Model file for the job. Use its own axes, mm. A direction names the side the tool comes from. Give positions to 0.01 mm unless a question says otherwise; leave off trailing zeros. Loops run counter-clockwise (first coordinate to the right, second up) from the corner with the lowest first, then second, coordinate; pieces in that order, holes last. Notation, with made-up numbers: (88.5, 11.5) - (112.5, 11.5) arc R31 cw to (112.5, 39.5) - close; hole circle Ø8 at (-14.5, 21.25). An arc over 180 degrees is marked (long way). Use a Markdown table: item, result.
Autodesk Inventor part; units mm, degrees
ref_plane "YZ Plane" through (0, 0, 0) normal (1, 0, 0) x (0, 1, 0)
ref_plane "XZ Plane" through (0, 0, 0) normal (0, 1, 0) x (-1, 0, 0)
ref_plane "XY Plane" through (0, 0, 0) normal (0, 0, 1) x (1, 0, 0)
sketch "Sketch1" plane through (0, 0, 0) normal (1, 0, 0) x (0, 1, 0)
  line L0 (0, 0) -> (-78.6, 0)
  line L1 (-78.6, 0) -> (-78.6, -45)
  line L2 (-78.6, -45) -> (0, -45)
  line L3 (0, -45) -> (0, 0)
  dimension "d0" = 78.6
  dimension "d1" = 45
extrude "Extrusion1" add sketch "Sketch1" along normal blind 20
sketch "Sketch2" plane through (20, 0, 0) normal (1, 0, 0) x (0, 0, -1)
  circle A0 centre (22.5, -27.8) radius 17.5
  line L0 (45, -78.6) -> (45, 0)
  line L1 (0, -78.6) -> (45, -78.6)
  point P0 (0, 0)
  dimension "d4" = 35
  dimension "d5" = 22.5
  dimension "d6" = 50.8
extrude "Extrusion2" add sketch "Sketch2" along normal blind 10
sketch "Sketch3" plane through (30, -27.8, -22.5) normal (1, 0, 0) x (0, 0, -1)
  circle A0 centre (0, 0) radius 3
  point P0 (-22.5, 27.8)
  dimension "d9" = 6
extrude "Extrusion3" add sketch "Sketch3" along normal blind 44
fillet "Fillet1" radius 5 2 edges at (10, 0, 0) (10, 0, -45)
sketch "Sketch4" plane through (0, 0, -5) normal (0, 1, 0) x (1, 0, 0)
  line L0 (6.488, 30) -> (2.488, 30)
  line L1 (2.488, 30) -> (2.488, 26)
  line L2 (2.488, 26) -> (6.488, 26)
  line L3 (6.488, 26) -> (6.488, 30)
  line L4 (6.488, 9) -> (2.488, 9)
  line L5 (2.488, 9) -> (2.488, 5)
  line L6 (2.488, 5) -> (6.488, 5)
  line L7 (6.488, 5) -> (6.488, 9)
  line L8 (0, 35) -> (20, 35)
  line L9 (20, 0) -> (0, 0)
  point P0 (0, -5)
  dimension "d13" = 4
  dimension "d14" = 4
  dimension "d15" = 4
  dimension "d16" = 4
  dimension "d17" = 5
  dimension "d18" = 9
extrude "Extrusion4" add sketch "Sketch4" along normal blind 5
chamfer "Chamfer1" distance 2 angle 45 1 edges at (30, -27.8, -5)
fillet "Fillet2" radius 5 5 edges at (20, -1.4645, -1.4645) (20, -41.8, 0) (20, -1.4645, -43.5355) (20, -41.8, -45) (20, 0, -22.5)
fillet "Fillet3" radius 2 1 edges at (74, -27.8, -19.5)
sketch "Sketch5" plane through (30, -27.8, -22.5) normal (1, 0, 0) x (0, 0, -1)
  point P0 (-22.5, 27.8)
properties part number "dc"
(1) Mould opens along Z. For faces 1 (the cylindrical face through (8, -2, -44)), 2 (the flat face through (4, 2, -10)), 3 (the flat face through (7, 0, -23)), 4 (the flat face through (6.488, 2, -12)) say: pulls with the +Z half, pulls with the -Z half, needs draft (parallel to the pull), parting line crosses it, or undercut.
Computed:
| item | result |
|---|---|
| face 1 | pulls with the -Z half |
| face 2 | pulls with the +Z half |
| face 3 | undercut |
| face 4 | needs draft |
(2) Slice it at A-A, the plane x = 58. Write the cut outline in (y, z), plus the area to 3 significant figures.
Computed:
| item | result |
|---|---|
| outline | circle Ø6 at (-27.8, -22.5) |
| area | 28.3 mm² |
(3) Pin check, flat tips, straight feed: P1, Ø4.5, axis at x = 6, z = -18, coming from the +Y side; P2, Ø2, axis at y = 1.5, z = -33, coming from the +X side; P3, Ø4.5, axis at x = 4.5, y = 3, coming from the +Z side. Stop position of each tip, or through.
Computed:
| item | result |
|---|---|
| P1 | y = 0 |
| P2 | x = 6.49 |
| P3 | z = -10 |
(4) 3-axis set-ups, long thin cutter, end or side, ignore diameter. For faces 5 (the flat face through (2.488, 2, -12)), 6 (the flat face through (5, 2, -35)), 7 (the flat face through (4, 2, -31)): which of +Z, -Z, +X, -X, +Y, -Y reach the whole face in a straight line?
Computed:
| item | result |
|---|---|
| face 5 | +Z, -Z, -X, +Y |
| face 6 | -Z, +X, -X, +Y |
| face 7 | +X, -X, +Y |
(5) Drill centre lines: probe 1 along Y at (x, z) = (13.5, -18.5); probe 2 along X at (y, z) = (-14.5, -34); probe 3 along X at (y, z) = (-32, -37). Where is each one in solid material? Low to high. Write a range as [from, to].
Computed:
| item | result |
|---|---|
| probe 1 | [-78.6, 0] |
| probe 2 | [0, 20] |
| probe 3 | [0, 30] |
